from build123d import *

# Parameters (mm, degrees)
SKETCH1_W           = 65
SKETCH1_H           = 40
SKETCH1_R           = 6.1
BOSS_EXTRUDE1_DEPTH = 19
SKETCH4_W           = 65
SKETCH4_H           = 14.8
BOSS_EXTRUDE2_DEPTH = 35
SKETCH6_W           = 10
SKETCH6_H           = 12
CUT_EXTRUDE1_DEPTH  = 71.109485806
CUT_EXTRUDE3_DEPTH  = 76.779284768
FILLET1_R           = 1
SKETCH9_W           = 65
SKETCH9_H           = 14.8
CUT_EXTRUDE4_DEPTH  = 5
SKETCH10_W          = 65
SKETCH10_H          = 14.8
CUT_EXTRUDE5_DEPTH  = 5
SKETCH11_R          = 2.6
CUT_EXTRUDE6_DEPTH  = 73.955465868
CUT_EXTRUDE7_DEPTH  = 10
CHAMFER1_SIZE       = 2
SKETCH13_W          = 14.3
SKETCH13_H          = 20
SKETCH13_R          = 1.2
BOSS_EXTRUDE3_DEPTH = 5


with BuildPart() as part:
    # Sketch1 → Boss-Extrude1 (new body)
    with BuildSketch(Plane.XY):
        with Locations((14, 7.8)):
            Rectangle(SKETCH1_W, SKETCH1_H)
        with Locations((-2, 0)):
            Circle(SKETCH1_R, mode=Mode.SUBTRACT)
        with Locations((30, 0)):
            Circle(SKETCH1_R, mode=Mode.SUBTRACT)
    extrude(amount=-BOSS_EXTRUDE1_DEPTH)

    # Sketch4 → Boss-Extrude2 (add, symmetric)
    with BuildSketch(Plane.XY.offset(-9.5)):
        with Locations((14, 20.4)):
            Rectangle(SKETCH4_W, SKETCH4_H)
    extrude(amount=BOSS_EXTRUDE2_DEPTH, both=True)

    # Sketch6 → Cut-Extrude1 (cut, through all)
    with BuildSketch(Plane.XY):
        with Locations((14, 7)):
            Rectangle(SKETCH6_W, SKETCH6_H)
    extrude(amount=-CUT_EXTRUDE1_DEPTH, mode=Mode.SUBTRACT)

    # Sketch8 → Cut-Extrude3 (cut, through all)
    with BuildSketch(Plane(origin=(0, 27.8, 0), x_dir=(1, 0, 0), z_dir=(0, 1, 0))):
        with BuildLine():
            Line((18, 29.5), (10, 29.5))
            ThreePointArc((10, 29.5), (7.5, 32), (10, 34.5))
            Line((10, 34.5), (18, 34.5))
            ThreePointArc((18, 34.5), (20.5, 32), (18, 29.5))
        make_face()
        with BuildLine():
            Line((18, -10.5), (10, -10.5))
            ThreePointArc((10, -10.5), (7.5, -13), (10, -15.5))
            Line((10, -15.5), (18, -15.5))
            ThreePointArc((18, -15.5), (20.5, -13), (18, -10.5))
        make_face()
    extrude(amount=-CUT_EXTRUDE3_DEPTH, mode=Mode.SUBTRACT)

    # Fillet1
    fillet1_edges = [part.edges().sort_by_distance(p)[0] for p in [
        (14, 1, -19),
        (9, 7, -19),
        (19, 7, -19),
        (9, 1, -9.5),
        (19, 1, -9.5),
        (9, 7, 0),
        (14, 1, 0),
        (19, 7, 0),
        (14, -12.2, 0),
        (46.5, -12.2, -9.5),
        (-18.5, -12.2, -9.5),
        (14, -12.2, -19),
    ]]
    fillet(fillet1_edges, radius=FILLET1_R)

    # Sketch9 → Cut-Extrude4 (cut)
    with BuildSketch(Plane.XY.offset(25.5)):
        with Locations((14, 20.4)):
            Rectangle(SKETCH9_W, SKETCH9_H)
    extrude(amount=-CUT_EXTRUDE4_DEPTH, mode=Mode.SUBTRACT)

    # Sketch10 → Cut-Extrude5 (cut)
    with BuildSketch(Plane(origin=(0, 0, -44.5), x_dir=(-1, 0, 0), z_dir=(0, 0, -1))):
        with Locations((-14, 20.4)):
            Rectangle(SKETCH10_W, SKETCH10_H)
    extrude(amount=-CUT_EXTRUDE5_DEPTH, mode=Mode.SUBTRACT)

    # Sketch11 → Cut-Extrude6 (cut, through all)
    with BuildSketch(Plane(origin=(0, 27.8, 0), x_dir=(1, 0, 0), z_dir=(0, 1, 0))):
        with Locations(Location((40.25, -14.25, 0), (0, 0, 270))):
            Circle(SKETCH11_R)
        with Locations(Location((40.25, 33.25, 0), (0, 0, 180))):
            Circle(SKETCH11_R)
        with Locations(Location((-12.25, 33.25, 0), (0, 0, 270))):
            Circle(SKETCH11_R)
        with Locations(Location((-12.25, -14.25, 0), (0, 0, 180))):
            Circle(SKETCH11_R)
    extrude(amount=-CUT_EXTRUDE6_DEPTH, mode=Mode.SUBTRACT)

    # Sketch12 → Cut-Extrude7 (cut)
    with BuildSketch(Plane.XZ.offset(-13)):
        with BuildLine():
            Line((-18.5, -39.5), (46.5, -39.5))
            Line((46.5, -39.5), (46.5, -19))
            Line((46.5, -19), (20, -19))
            ThreePointArc((20, -19), (19.292893219, -18.707106781), (19, -18))
            Line((19, -18), (19, -1))
            ThreePointArc((19, -1), (19.292893219, -0.292893219), (20, 0))
            Line((20, 0), (46.5, 0))
            Line((46.5, 0), (46.5, 20.5))
            Line((46.5, 20.5), (-18.5, 20.5))
            Line((-18.5, 20.5), (-18.5, 0))
            Line((-18.5, 0), (8, 0))
            ThreePointArc((8, 0), (8.707106781, -0.292893219), (9, -1))
            Line((9, -1), (9, -18))
            ThreePointArc((9, -18), (8.707106781, -18.707106781), (8, -19))
            Line((8, -19), (-18.5, -19))
            Line((-18.5, -19), (-18.5, -39.5))
        make_face()
    extrude(amount=-CUT_EXTRUDE7_DEPTH, mode=Mode.SUBTRACT)

    # Chamfer1
    chamfer1_edges = [part.edges().sort_by_distance(p)[0] for p in [
        (-5.25, 23, -19),
        (8.707106781, 23, -18.707106781),
        (9, 23, -9.5),
        (8.707106781, 23, -0.292893219),
        (-5.25, 23, 0),
        (33.25, 23, 0),
        (19.292893219, 23, -0.292893219),
        (19, 23, -9.5),
        (19.292893219, 23, -18.707106781),
        (33.25, 23, -19),
    ]]
    chamfer(chamfer1_edges, length=CHAMFER1_SIZE)

    # Sketch13 → Boss-Extrude3 (add)
    with BuildSketch(Plane(origin=(46.5, 0, 0), x_dir=(0, 0, -1), z_dir=(1, 0, 0))):
        with Locations((26.15, -2.2)):
            Rectangle(SKETCH13_W, SKETCH13_H)
        with Locations((25.4, 2.55)):
            Circle(SKETCH13_R, mode=Mode.SUBTRACT)
        with Locations((25.4, -7.05)):
            Circle(SKETCH13_R, mode=Mode.SUBTRACT)
    extrude(amount=-BOSS_EXTRUDE3_DEPTH)


solid = part.part
CAD build for the part. Positions are in the model's coordinates, mm. A direction names the side the tool comes from. Round coordinates to 2 decimals unless told otherwise and drop trailing zeros. Order: outer loops, then holes, each group sorted by start corner. A loop starts at its lowest first (then second) coordinate and runs counter-clockwise, first axis right, second up. Notation, with made-up numbers: (71, -20) - (99, -20) arc R20 cw to (99, 11) - close; hole circle Ø8 at (67, 9). An arc over 180 degrees is marked (long way). Return JSON: item names as keys, results as strings.
(1) Pull direction Z, two halves, no side cores. Call faces 1 (the face through (-13.832, 25.434, -35.313)), 2 (the face through (19, 11, -10)), 3 (the face through (18.58, 21.986, 0.389)), 4 (the face through (44.04, -7.51, -26.51)): +Z half, -Z half, draft (parallel to the pull), parting line (faces both ways), or undercut.
Answer key:
{"face 1": "undercut", "face 2": "draft", "face 3": "+Z half", "face 4": "undercut"}
(2) Cut at C-C (z = -7.5). Give the cut face in (x, y).
Answer key:
{"outline": "(-18.5, -11.2) arc R1 ccw to (-17.5, -12.2) - (45.5, -12.2) arc R1 ccw to (46.5, -11.2) - (46.5, 27.8) - (-18.5, 27.8) - close; hole circle Ø12.2 at (-2, 0); hole (9, 2) arc R1 ccw to (10, 1) - (18, 1) arc R1 ccw to (19, 2) - (19, 21) - (17, 23) - (11, 23) - (9, 21) - close; hole circle Ø12.2 at (30, 0)"}
(3) Wall check: probe 1 along Y at (x, z) = (45.55, -25.4); probe 2 along Z at (x, y) = (40, 25); probe 3 along Z at (x, y) = (43, -7). Give the ranges that are in metal, low to high. Write a range as from..to.
Answer key:
{"probe 1": "y = -12.2..-8.25, -5.85..1.35, 3.75..7.8, 23..27.8", "probe 2": "z = -39.5..-35.84, -30.66..11.66, 16.84..20.5", "probe 3": "z = -33.3..-26.6, -24.2..0"}
(4) Cut at B-B (y = 19). Give the cut face in (x, z).
Answer key:
{"outline": "(-18.5, -19) - (8, -19) arc R1 ccw to (9, -18) - (9, -1) arc R1 ccw to (8, 0) - (-18.5, 0) - close; (19, -18) arc R1 ccw to (20, -19) - (46.5, -19) - (46.5, 0) - (20, 0) arc R1 ccw to (19, -1) - close"}
(5) Cut at D-D (x = 30). Give the cut face in (y, z), then the cut area to 3 significant figures.
Answer key:
{"outline": "(-12.2, -18) arc R1 ccw to (-11.2, -19) - (-6.1, -19) - (-6.1, 0) - (-11.2, 0) arc R1 ccw to (-12.2, -1) - close; (6.1, -19) - (21, -19) - (23, -21) - (23, -39.5) - (27.8, -39.5) - (27.8, 20.5) - (23, 20.5) - (23, 2) - (21, 0) - (6.1, 0) - close", "area": "729 mm^2"}
(6) Tool access for faces 5 (the face through (20.5, 25.4, -32.1)), 6 (the face through (33, 22, -20)), 7 (the face through (18, 22, -10)), 8 (the face through (6, 5, 0)), 9 (the face through (14, 27.8, -9)): list every direction of +Z, -Z, +X, -X, +Y, -Y with a clear straight run to the whole face (end or side of a thin tool).
Answer key:
{"face 5": "+Y, -Y", "face 6": "-Z, +X, -X", "face 7": "+Z, -Z", "face 8": "+Z, +X, -X, -Y", "face 9": "+Z, -Z, +X, -X, +Y"}
(7) Cut at A-A (x = 15.5). Give the cut face in (y, z), then the cut area to 3 significant figures.
Answer key:
{"outline": "(-12.2, -18) arc R1 ccw to (-11.2, -19) - (0, -19) arc R1 ccw to (1, -18) - (1, -1) arc R1 ccw to (0, 0) - (-11.2, 0) arc R1 ccw to (-12.2, -1) - close; (23, -39.5) - (27.8, -39.5) - (27.8, -34.5) - (23, -34.5) - close; (23, -29.5) - (27.8, -29.5) - (27.8, 10.5) - (23, 10.5) - close; (23, 15.5) - (27.8, 15.5) - (27.8, 20.5) - (23, 20.5) - close", "area": "490 mm^2"}
(8) Pin check, flat tips, straight feed: pin 1 Ø0.8 at (x, y) = (44.5, -12) entering from +Z; pin 2 Ø1 at (x, y) = (-6.5, 19) entering from +Z; pin 3 Ø1 at (x, y) = (25.5, 21) entering from -Z. Stop position of each tip, or through.
Answer key:
{"pin 1": "stops at z = -0.08", "pin 2": "stops at z = 0", "pin 3": "stops at z = -19.5"}
